The model under review builds one solid part; all positions refer to its coordinate system, in mm. Face numbers are marked on the shaded views. A direction names the side the tool comes from. Round coordinates to 2 decimals unless told otherwise and drop trailing zeros. Order: outer loops, then holes, each group sorted by start corner. A loop starts at its lowest first (then second) coordinate and runs counter-clockwise, first axis right, second up.
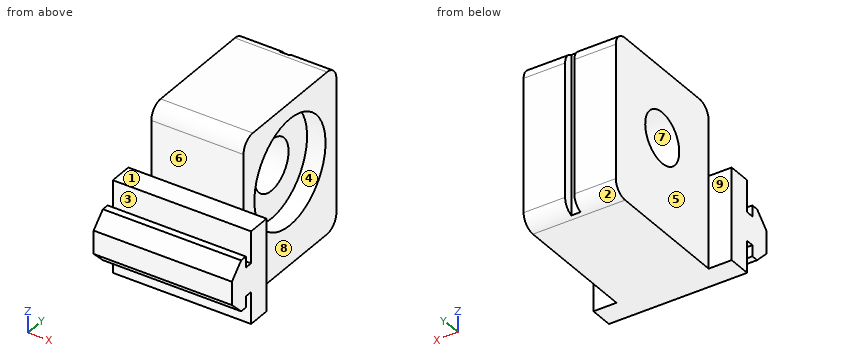
Autodesk Fusion 360 part; units mm, degrees
sketch "Sketch1" plane through (0, 0, 0) normal (1, 0, 0) x (0, 0, -1)
  line L0 (0, 0) -> (2.5225, 0)
  line L1 (2.5225, 0) -> (5.5, 2.98)
  line L2 (5.5, 2.98) -> (5.5, 4.5)
  line L3 (5.5, 4.5) -> (3.1, 4.5)
  line L4 (3.1, 4.5) -> (3.1, 6.2)
  line L5 (3.1, 6.2) -> (10, 6.2)
  line L6 (10, 6.2) -> (10, 11.2)
  line L7 (10, 11.2) -> (0, 11.2)
  line L8 (0, 0) -> (0, 21.3117) construction
  line L9 (-10, 6.2) -> (-10, 11.2)
  line L10 (0, 0) -> (-2.5225, 0)
  line L11 (-3.1, 6.2) -> (-10, 6.2)
  line L12 (-5.5, 2.98) -> (-5.5, 4.5)
  line L13 (-10, 11.2) -> (0, 11.2)
  line L14 (-5.5, 4.5) -> (-3.1, 4.5)
  line L15 (-2.5225, 0) -> (-5.5, 2.98)
  line L16 (-3.1, 4.5) -> (-3.1, 6.2)
  dimension "d3" = 2.5225
  dimension "d4" = 4.5
  dimension "d6" = 2.4
  dimension "d7" = 3.1
  dimension "d8" = 1.52
  dimension "d9" = 1.7
  dimension "d10" = 5
  dimension "d11" = 10
extrude "Extrude1" add sketch "Sketch1" along normal blind 30
ref_plane "WorkPlane1" through (15, 5.6, 0) normal (1, 0, 0) x (0, 0, -1)
sketch "Sketch2" plane through (15, 5.6, 0) normal (1, 0, 0) x (0, 0, -1)
  line L0 (10, 5.6) -> (-10, 5.6)
  line L1 (10, 5.6) -> (-22, 5.6)
  line L2 (-25, 8.6) -> (-25, 32.6)
  line L3 (-22, 35.6) -> (7, 35.6)
  line L4 (10, 32.6) -> (10, 5.6)
  circle A0 centre (-10, 20.6) radius 11.5
  line L5 (-25, 20.6) -> (10, 20.6) construction
  circle A1 centre (-10, 20.6) radius 5.5
  arc A2 (-22, 35.6) -> (-25, 32.6) centre (-22, 32.6) ccw
  arc A3 (10, 32.6) -> (7, 35.6) centre (7, 32.6) ccw
  arc A4 (-25, 8.6) -> (-22, 5.6) centre (-22, 8.6) ccw
  point P0 (-25, 5.6)
  point P1 (10, 35.6)
  dimension "d15" = 35
  dimension "d16" = 30
  dimension "d17" = 23
  dimension "d18" = 15
  dimension "d19" = 11
  dimension "d29" = 3
  dimension "d30" = 3
extrude "Extrude2" add sketch "Sketch2" along normal blind 10 and the other way blind 10 contours L0 L1 L2 L3 L4 A2 A3 A4
extrude "Extrude3" add sketch "Sketch2" against normal blind 10 and the other way blind 6 contours A0
sketch "Sketch3" plane through (0, 0, 25) normal (0, 0, 1) x (1, 0, 0)
  line L0 (5, 14.2) -> (25, 14.2)
  line L1 (25, 14.2) -> (25, 38.2)
  line L2 (25, 38.2) -> (5, 38.2)
  line L3 (5, 38.2) -> (5, 14.2)
  line L4 (25, 41.2) -> (5, 41.2)
  line L5 (14, 41.2) -> (16, 41.2)
  line L6 (16, 41.2) -> (16, 39.2)
  line L7 (16, 39.2) -> (14, 39.2)
  line L8 (14, 39.2) -> (14, 41.2)
  dimension "d31" = 2
  dimension "d32" = 2
extrude "Extrude4" cut sketch "Sketch3" against normal through all contours L4 L5 L6 L7 L8
(1) We need section C-C (x = 27). Give the boundary of the cut face in (y, z).
(2) The part is to be moulded in two halves that separate along Y. For the marked faces 6, 7, 8 and 9, say which applies: pulls with the +Y half, pulls with the -Y half, needs draft (parallel to the pull), parting line crosses it, or undercut.
(3) To check wall thickness, follow L1, parallel to Y at x = 2.75, z = 6.5; L2, parallel to Y at x = 26.75, z = 0; L3, parallel to X at y = 17.5, z = 12. State the ranges of each line that lie inside material, in increasing order.
(4) We need section B-B (x = 21.75). Give the boundary of the cut face in (y, z).
(5) Clearance check with flat-ended pins moving along their axes: P1, Ø0.5, axis at x = 22, y = 4, coming from the -Z side; P2, Ø2, axis at y = 40, z = 3.5, coming from the -X side; P3, Ø0.8, axis at x = 22, y = 5.5, coming from the +Z side. State where each tip first meets the part, or that it passes through.
(6) Tool access review of the marked faces 1, 2, 3, 4 and 5: name each direction out of +Z, -Z, +X, -X, +Y, -Y from which nothing blocks a thin tool from reaching the whole face with its end or side.
(7) We need section A-A (y = 26.2). Give the boundary of the cut face in (x, z).
(8) We need section D-D (x = 8). Give the boundary of the cut face in (y, z), and give its area (3 significant figures).
Verdict:
1. outline: (0, -2.52) - (2.98, -5.5) - (4.5, -5.5) - (4.5, -3.1) - (6.2, -3.1) - (6.2, -10) - (11.2, -10) - (11.2, 10) - (6.2, 10) - (6.2, 3.1) - (4.5, 3.1) - (4.5, 5.5) - (2.98, 5.5) - (0, 2.52) - close
2. face 6: pulls with the -Y half
2. face 7: undercut
2. face 8: needs draft
2. face 9: pulls with the +Y half
3. L1: y = 6.2 to 11.2
3. L2: y = 0 to 11.2
3. L3: x = 5 to 21
4. outline: (0, -2.52) - (2.98, -5.5) - (4.5, -5.5) - (4.5, -3.1) - (6.2, -3.1) - (6.2, -10) - (38.2, -10) arc R3 ccw to (41.2, -7) - (41.2, 22) arc R3 ccw to (38.2, 25) - (14.2, 25) arc R3 ccw to (11.2, 22) - (11.2, 10) - (6.2, 10) - (6.2, 3.1) - (4.5, 3.1) - (4.5, 5.5) - (2.98, 5.5) - (0, 2.52) - close; hole circle Ø23 at (26.2, 10)
5. P1: stops at z = -5.5
5. P2: stops at x = 5
5. P3: stops at z = 3.1
6. face 1: +Z, +X, -X, -Y
6. face 2: -Z, +X, -X, +Y
6. face 3: +Z, +X, -X
6. face 4: +X
6. face 5: +Z, -Z, -X, +Y
7. outline: (5, -10) - (25, -10) - (25, -1.5) - (21, -1.5) - (21, 4.5) - (5, 4.5) - close; (5, 15.5) - (21, 15.5) - (21, 21.5) - (25, 21.5) - (25, 25) - (5, 25) - close
8. outline: (0, -2.52) - (2.98, -5.5) - (4.5, -5.5) - (4.5, -3.1) - (6.2, -3.1) - (6.2, -10) - (38.2, -10) arc R3 ccw to (41.2, -7) - (41.2, 22) arc R3 ccw to (38.2, 25) - (14.2, 25) arc R3 ccw to (11.2, 22) - (11.2, 10) - (6.2, 10) - (6.2, 3.1) - (4.5, 3.1) - (4.5, 5.5) - (2.98, 5.5) - (0, 2.52) - close; hole circle Ø11 at (26.2, 10)
8. area: 1,100 mm2
